Input: part model. Units: mm. Frame: model coordinates. A direction names the side the tool comes from. Give positions to 0.01 mm unless a question says otherwise; leave off trailing zeros. Write each loop counter-clockwise with the first axis right and the second up, starting at its lowest first coordinate (ties: lowest second). Pieces come first, ordered by that corner, then holes. Notation, with made-up numbers: (-25, -24) -> (32, -24) arc R17 cw to (32, -8) -> close; hole circle Ø3 at (74, 18). An arc over 180 degrees is marked (long way). Return JSON: item names as keys, results as strings. Group by question number.
Item 1: Pin query (flat end, axial travel): P1, Ø8, axis at y = 5.5, z = -10.5, coming from the -X side; P2, Ø2, axis at y = 13.5, z = -11, coming from the +X side; P3, Ø2, axis at x = -10.5, z = 2.5, coming from the +Y side. Return the tip coordinate at first contact, or that it passes through.
Item 2: Section B-B, the plane y = 23. Return loops of the section in (x, z), then the cut area to 3 significant figures.
Item 3: Section A-A, the plane y = 19. Return loops of the section in (x, z).
Item 4: Line query: line 1 (Y direction, x = 0, z = 12.25); line 2 (X direction, y = 10.5, z = 8.5); line 3 (Y direction, x = 5, z = 7). Output: solid intervals per line, ascending. Write a range as [from, to].
Item 5: Set-up query: faces 1 (the face through (-10.781, 18, -9)), 2 (the face through (11.837, 17, -9)), 3 (the face through (1, 18, 8)). Return all of +Z, -Z, +X, -X, +Y, -Y with unobstructed straight access to the full face (end or side cutting, diameter ignored); none if empty.
Item 6: Section C-C, the plane x = -1.5. Return loops of the section in (y, z).
Item 7: Mould query, pull axis Y, two halves, no side actions, for faces 4 (the face through (-1.559, 22.003, 11.549)), 5 (the face through (0.44, 28.35, -11.45)), 6 (the face through (0.717, 31.255, 10.774)), 7 (the face through (-10.781, 18, 9)). Classes: released by +Y, released by -Y, zero draft, split by the parting line, or undercut.
Item 8: Section D-D, the plane z = -10. Return loops of the section in (x, y).
from build123d import *

# Parameters (mm, degrees)
SKETCH1_R                            = 15
BOSS_EXTRUDE1_DEPTH                  = 10
BOSS_EXTRUDE2_REACH                  = 25.452
BOSS_EXTRUDE2_END_RADIUS             = 15
BOSS_EXTRUDE2_DIRECTION_2_REACH      = 25.452
BOSS_EXTRUDE2_DIRECTION_2_END_RADIUS = 15
SKETCH3_W                            = 16
SKETCH3_H                            = 50
CUT_EXTRUDE1_DEPTH                   = 44.842776862
CUT_EXTRUDE2_DEPTH                   = 42.60493807
CUT_EXTRUDE2_DEPTH_BACK              = 42.60493807
SKETCH4_R                            = 3.3782


with BuildPart() as part:
    # Sketch1 → Boss-Extrude1 (new body)
    with BuildSketch(Plane(origin=(0, 0, 0), x_dir=(1, 0, 0), z_dir=(0, 1, 0))):
        with Locations(Location((0, 0, 0), (0, 0, 270))):
            Circle(SKETCH1_R)
    extrude(amount=BOSS_EXTRUDE1_DEPTH)

    # Boss-Extrude2: up to this cylinder (the profile starts inside it)
    boss_extrude2_end = Plane(origin=(0, 19.788333, 0), z_dir=(0, -1, 0)) * Cylinder(BOSS_EXTRUDE2_END_RADIUS, 81.904, mode=Mode.PRIVATE)
    # Sketch2 → Boss-Extrude2 (add, up to the surface)
    with BuildSketch(Plane.XY, mode=Mode.PRIVATE) as boss_extrude2_sk1:
        with BuildLine():
            Line((-10.780802974, 10), (11.836881633, 10))
            Line((11.836881633, 10), (11.836881633, 25))
            ThreePointArc((11.836881633, 25), (0.528039329, 31.256533044), (-10.780802974, 25))
            Line((-10.780802974, 25), (-10.780802974, 10))
        make_face()
    boss_extrude2_tool1 = extrude(boss_extrude2_sk1.sketch, amount=BOSS_EXTRUDE2_REACH, mode=Mode.PRIVATE) & boss_extrude2_end
    add(boss_extrude2_tool1.solids().sort_by_distance((0.528039, 19.788333, 0))[0])

    # Boss-Extrude2 direction 2: up to this cylinder (the profile starts inside it)
    boss_extrude2_direction_2_end = Plane(origin=(0, 19.788333, 0), z_dir=(0, -1, 0)) * Cylinder(BOSS_EXTRUDE2_DIRECTION_2_END_RADIUS, 81.904, mode=Mode.PRIVATE)
    # Sketch2 → Boss-Extrude2 direction 2 (add, up to the surface)
    with BuildSketch(Plane.XY, mode=Mode.PRIVATE) as boss_extrude2_direction_2_sk1:
        with BuildLine():
            Line((-10.780802974, 10), (11.836881633, 10))
            Line((11.836881633, 10), (11.836881633, 25))
            ThreePointArc((11.836881633, 25), (0.528039329, 31.256533044), (-10.780802974, 25))
            Line((-10.780802974, 25), (-10.780802974, 10))
        make_face()
    boss_extrude2_direction_2_tool1 = extrude(boss_extrude2_direction_2_sk1.sketch, amount=-BOSS_EXTRUDE2_DIRECTION_2_REACH, mode=Mode.PRIVATE) & boss_extrude2_direction_2_end
    add(boss_extrude2_direction_2_tool1.solids().sort_by_distance((0.528039, 19.788333, 0))[0])

    # Sketch3 → Cut-Extrude1 (cut, through all)
    with BuildSketch(Plane(origin=(11.836881633, 0, 0), x_dir=(0, 0, -1), z_dir=(1, 0, 0))):
        with Locations((0, 35)):
            Rectangle(SKETCH3_W, SKETCH3_H)
    extrude(amount=-CUT_EXTRUDE1_DEPTH, mode=Mode.SUBTRACT)

    # Sketch4 → Cut-Extrude2 (cut, two sides: drawn at the far end of the back side and taken through both)
    with BuildSketch(Plane(origin=(0, 0, 8), x_dir=(-1, 0, 0), z_dir=(0, 0, -1)).offset(-CUT_EXTRUDE2_DEPTH_BACK)):
        with Locations((0, 25)):
            Circle(SKETCH4_R)
    extrude(amount=CUT_EXTRUDE2_DEPTH + CUT_EXTRUDE2_DEPTH_BACK, mode=Mode.SUBTRACT)


solid = part.part
Answer below:
{
 "1": {"P1": "stops at x = -13.52", "P2": "stops at x = 11.18", "P3": "stops at y = 10"},
 "2": {"outline": "(-10.78, -10.43) arc R15 ccw to (-2.72, -14.75) -> (-2.72, -8) -> (-10.78, -8) -> close; (-10.78, 8) -> (-2.72, 8) -> (-2.72, 14.75) arc R15 ccw to (-10.78, 10.43) -> close; (2.72, -14.75) arc R15 ccw to (11.84, -9.21) -> (11.84, -8) -> (2.72, -8) -> close; (2.72, 8) -> (11.84, 8) -> (11.84, 9.21) arc R15 ccw to (2.72, 14.75) -> close", "area": "169 mm2"},
 "3": {"outline": "(-10.78, -10.43) arc R15 ccw to (11.84, -9.21) -> (11.84, -8) -> (-10.78, -8) -> close; (-10.78, 8) -> (11.84, 8) -> (11.84, 9.21) arc R15 ccw to (-10.78, 10.43) -> close"},
 "4": {"line 1": "y = [0, 21.62], [28.38, 31.25]", "line 2": "x = [-10.78, 11.84]", "line 3": "y = [0, 10]"},
 "5": {"face 1": "+Z, -Z, -X, +Y", "face 2": "+Z, -Z, +X, +Y", "face 3": "+X, -X, +Y"},
 "6": {"outline": "(0, -14.92) -> (21.97, -14.92) -> (21.97, -8) -> (10, -8) -> (10, 8) -> (21.97, 8) -> (21.97, 14.92) -> (0, 14.92) -> close; (28.03, -14.92) -> (31.1, -14.92) -> (31.1, -8) -> (28.03, -8) -> close; (28.03, 8) -> (31.1, 8) -> (31.1, 14.92) -> (28.03, 14.92) -> close"},
 "7": {"face 4": "undercut", "face 5": "undercut", "face 6": "released by +Y", "face 7": "zero draft"},
 "8": {"outline": "(-11.18, 0) -> (11.18, 0) -> (11.18, 25.95) arc R13.35 ccw to (-10.78, 25) -> (-10.78, 10) -> (-11.18, 10) -> close; hole circle Ø6.76 at (0, 25)"}
}
